Check sheet for the modelled part. Datum: model origin and axes. Units: mm. A direction names the side the tool comes from. Round coordinates to 2 decimals unless told otherwise and drop trailing zeros. Write each loop counter-clockwise with the first axis right and the second up, starting at its lowest first coordinate (ties: lowest second). Pieces come first, ordered by that corner, then holes.
Item 1: Section check C-C, the plane z = 1.75. Record the cut outline in (x, y), plus the area to 3 significant figures.
Item 2: Section check A-A, the plane x = 48. Record the cut outline in (y, z).
Item 3: Section check D-D, the plane y = -9. Record the cut outline in (x, z), plus the area to 3 significant figures.
Item 4: Material ranges on line 1 along Y through (x, z) = (53, 4.3); line 2 along X through (y, z) = (46.5, 2.8); line 3 along Y through (x, z) = (19, 3.4), recorded low to high.
Item 5: Release check for a two-part mould opening along X. For faces 4 (the flat face through (12, 30, 2)), 5 (the cylindrical face through (21.35, 13.09, 2.37)), 6 (the flat face through (61, 31, 2)) record: pulls with the +X half, pulls with the -X half, needs draft (parallel to the pull), parting line crosses it, or undercut.
Item 6: Depth check by flat-ended pin: pin 1 (3.5 mm diameter, centred on x = 52, y = 14.65, fed in from -Z); pin 2 (8 mm diameter, centred on x = 47, y = 27.5, fed in from -Z). Enter the tip coordinate at first touch or a pass-through.
Item 7: Set-up check for faces 1 (the flat face through (53, 2.65, 2)), 2 (the flat face through (27, -7, 2)), 3 (the cylindrical face through (50.52, 14.04, 2.37)): record each of +Z, -Z, +X, -X, +Y, -Y from which the full face is reachable in a straight line by a thin tool's end or side.
Item 8: Section check B-B, the plane y = 38. Record the cut outline in (x, z), plus the area to 3 significant figures.
from build123d import *

# Parameters (mm, degrees)
ESQUISSE1_R        = 15.75
ESQUISSE1_R_2      = 1.6
ESQUISSE1_R_3      = 1.35
BOSS_EXTRU_1_DEPTH = 4.8


with BuildPart() as part:
    # Esquisse1 → Boss.-Extru.1 (new body)
    with BuildSketch(Plane(origin=(0, 0, 0), x_dir=(-1, 0, 0), z_dir=(0, 0, -1))):
        with BuildLine():
            Line((-12.0004012, 3.650219609), (-12.0004012, 56.650219609))
            ThreePointArc((-12.0004012, 56.650219609), (-12.293294419, 57.35732639), (-13.0004012, 57.650219609))
            Line((-13.0004012, 57.650219609), (-60.0004012, 57.650219609))
            ThreePointArc((-60.0004012, 57.650219609), (-60.707507981, 57.35732639), (-61.0004012, 56.650219609))
            Line((-61.0004012, 56.650219609), (-61.0004012, 3.650219609))
            ThreePointArc((-61.0004012, 3.650219609), (-60.707507981, 2.943112828), (-60.0004012, 2.650219609))
            Line((-60.0004012, 2.650219609), (-46.0004012, 2.650219609))
            Line((-46.0004012, 2.650219609), (-46.0004012, -17.349780391))
            ThreePointArc((-46.0004012, -17.349780391), (-45.707507981, -18.056887172), (-45.0004012, -18.349780391))
            Line((-45.0004012, -18.349780391), (-28.0004012, -18.349780391))
            ThreePointArc((-28.0004012, -18.349780391), (-27.293294419, -18.056887172), (-27.0004012, -17.349780391))
            Line((-27.0004012, -17.349780391), (-27.0004012, 2.650219609))
            Line((-27.0004012, 2.650219609), (-13.0004012, 2.650219609))
            ThreePointArc((-13.0004012, 2.650219609), (-12.293294419, 2.943112828), (-12.0004012, 3.650219609))
        make_face()
        with Locations((-36.5004012, 30.150219609)):
            Circle(ESQUISSE1_R, mode=Mode.SUBTRACT)
        with Locations((-52.0004012, 14.650219609)):
            Circle(ESQUISSE1_R_2, mode=Mode.SUBTRACT)
        with Locations((-52.000444233, 45.650219609)):
            Circle(ESQUISSE1_R_2, mode=Mode.SUBTRACT)
        with Locations((-21.0004012, 14.650219609)):
            Circle(ESQUISSE1_R_2, mode=Mode.SUBTRACT)
        with Locations((-21.0004012, 45.650219609)):
            Circle(ESQUISSE1_R_2, mode=Mode.SUBTRACT)
        with Locations((-43.5004012, -15.849780391)):
            Circle(ESQUISSE1_R_3, mode=Mode.SUBTRACT)
        with Locations((-33.5004012, -15.849780391)):
            Circle(ESQUISSE1_R_3, mode=Mode.SUBTRACT)
    extrude(amount=-BOSS_EXTRU_1_DEPTH)


solid = part.part
Values found:
1. outline: (12, 3.65) arc R1 ccw to (13, 2.65) - (27, 2.65) - (27, -17.35) arc R1 ccw to (28, -18.35) - (45, -18.35) arc R1 ccw to (46, -17.35) - (46, 2.65) - (60, 2.65) arc R1 ccw to (61, 3.65) - (61, 56.65) arc R1 ccw to (60, 57.65) - (13, 57.65) arc R1 ccw to (12, 56.65) - close; hole circle Ø3.2 at (21, 14.65); hole circle Ø3.2 at (21, 45.65); hole circle Ø31.5 at (36.5, 30.15); hole circle Ø2.7 at (33.5, -15.85); hole circle Ø2.7 at (43.5, -15.85); hole circle Ø3.2 at (52, 14.65); hole circle Ø3.2 at (52, 45.65)
1. area: 2,270 mm2
2. outline: (2.65, 0) - (19.39, 0) - (19.39, 4.8) - (2.65, 4.8) - close; (40.91, 0) - (57.65, 0) - (57.65, 4.8) - (40.91, 4.8) - close
3. outline: (27, 0) - (46, 0) - (46, 4.8) - (27, 4.8) - close
3. area: 91.2 mm2
4. line 1: y = 2.65 to 13.4, 15.9 to 44.4, 46.9 to 57.65
4. line 2: x = 12 to 19.64, 22.36 to 50.64, 53.36 to 61
4. line 3: y = 2.65 to 57.65
5. face 4: pulls with the -X half
5. face 5: undercut
5. face 6: pulls with the +X half
6. pin 1: stops at z = 0
6. pin 2: passes through
7. face 1: +Z, -Z, +X, -Y
7. face 2: +Z, -Z, -X, -Y
7. face 3: +Z, -Z
8. outline: (12, 0) - (22.85, 0) - (22.85, 4.8) - (12, 4.8) - close; (50.15, 0) - (61, 0) - (61, 4.8) - (50.15, 4.8) - close
8. area: 104 mm2
